Source: three-view drawing plus pictorial views. Frame: mm from the lowest corner of the part. Give positions to 0.01 mm unless a question says otherwise; leave off trailing zeros. Write each loop counter-clockwise with the first axis right and the second up, starting at its lowest first coordinate (ties: lowest second). Pieces come first, ordered by that corner, then holes. Notation, with made-up numbers: (64, 40.25) -> (120, 40.25) arc R20 cw to (120, 63.25) -> close; hole circle Ø8 at (64.25, -16.75). An arc over 180 degrees is marked (long way). Use a Markdown table: item, result. Add a question column.
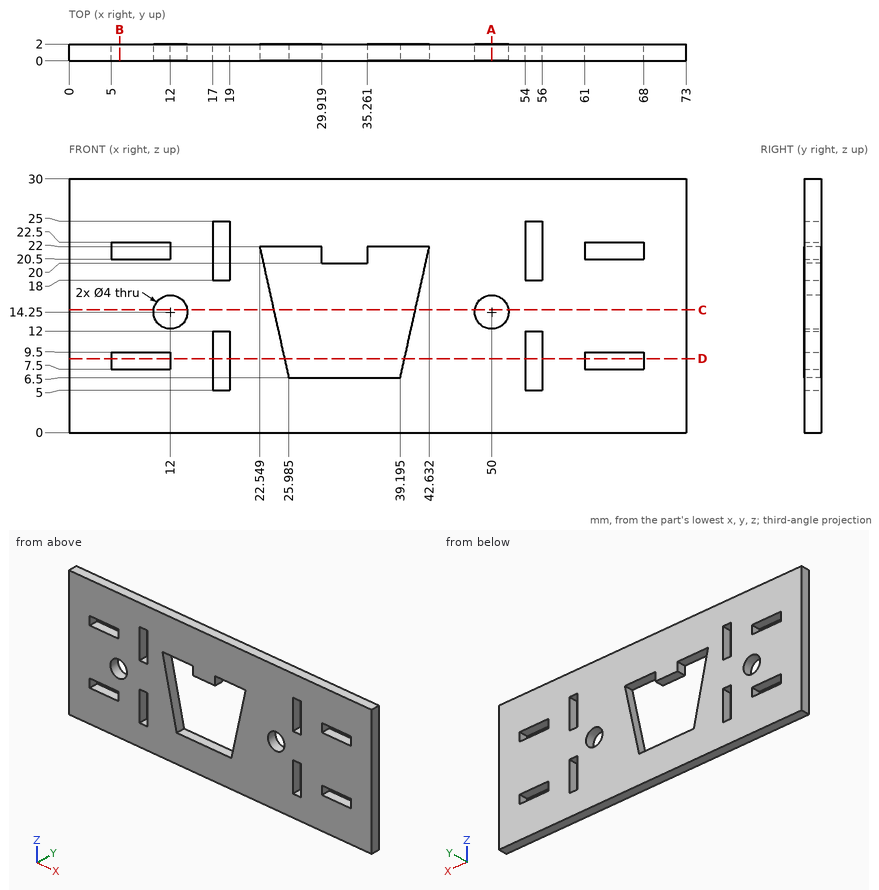
(1) Material intervals for L1, parallel to X at y = 0.55, z = 23.5; L2, parallel to X at y = 1.1, z = 14.25; L3, parallel to X at y = 0.25, z = 14.75 (1 decimal), sorted ascending.
(2) Cut plane D-D on z = 8.75. Return the cut outline in (x, y).
(3) Cut plane A-A on x = 50. Return the cut outline in (y, z).
(4) Cut plane C-C on z = 14.5. Return the cut outline in (x, y) (1 decimal).
(5) Cut plane B-B on x = 6. Return the cut outline in (y, z).
(6) First-contact query: pin 1 Ø3 at (x, z) = (50, 14.25) entering from +Y. Flat tip, straight axial feed; report the tip coordinate or a pass-through.
Output:
| question | item | result |
|---|---|---|
| 1 | L1 | 0 to 17, 19 to 54, 56 to 73 |
| 1 | L2 | 0 to 10, 14 to 24.27, 40.91 to 48, 52 to 73 |
| 1 | L3 | 0 to 10.1, 13.9 to 24.2, 41 to 48.1, 51.9 to 73 |
| 2 | outline | (0, 0) -> (5, 0) -> (5, 2) -> (0, 2) -> close; (12, 0) -> (17, 0) -> (17, 2) -> (12, 2) -> close; (19, 0) -> (25.49, 0) -> (25.49, 2) -> (19, 2) -> close; (39.69, 0) -> (54, 0) -> (54, 2) -> (39.69, 2) -> close; (56, 0) -> (61, 0) -> (61, 2) -> (56, 2) -> close; (68, 0) -> (73, 0) -> (73, 2) -> (68, 2) -> close |
| 3 | outline | (0, 0) -> (2, 0) -> (2, 12.25) -> (0, 12.25) -> close; (0, 16.25) -> (2, 16.25) -> (2, 30) -> (0, 30) -> close |
| 4 | outline | (0, 0) -> (10, 0) -> (10, 2) -> (0, 2) -> close; (14, 0) -> (24.2, 0) -> (24.2, 2) -> (14, 2) -> close; (41, 0) -> (48, 0) -> (48, 2) -> (41, 2) -> close; (52, 0) -> (73, 0) -> (73, 2) -> (52, 2) -> close |
| 5 | outline | (0, 0) -> (2, 0) -> (2, 7.5) -> (0, 7.5) -> close; (0, 9.5) -> (2, 9.5) -> (2, 20.5) -> (0, 20.5) -> close; (0, 22.5) -> (2, 22.5) -> (2, 30) -> (0, 30) -> close |
| 6 | pin 1 | through |
